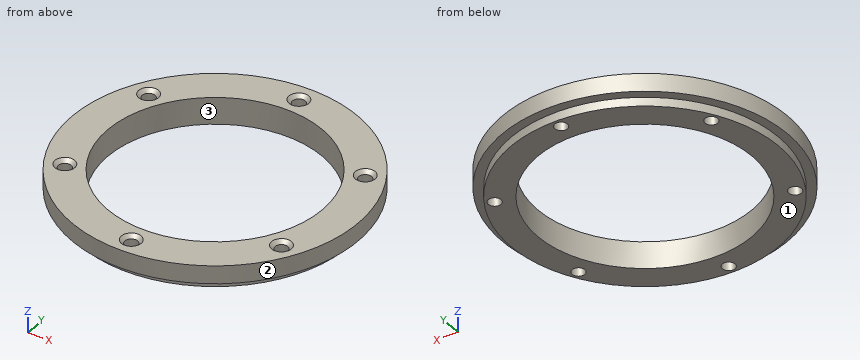
```python
from build123d import *

# Parameters (mm, degrees)
SKETCH1_R                       = 25.4
SKETCH1_R_2                     = 19.05
BOSS_EXTRUDE1_DEPTH             = 4.7625
F_4_40_TAPPED_HOLE1_D           = 2.2606
F_4_40_TAPPED_HOLE1_DEPTH       = 7.62
F_4_40_TAPPED_HOLE1_CSINK_D     = 3.5306
F_4_40_TAPPED_HOLE1_CSINK_ANGLE = 90
F_4_40_TAPPED_HOLE1_TIP         = 0.679152758
SKETCH5_OUTSIDE_W               = 67.2
SKETCH5_OUTSIDE_H               = 67.2
SKETCH5_OUTSIDE_R               = 23.8125
CUT_EXTRUDE1_DEPTH              = 1.5748


with BuildPart() as part:
    # Sketch1 → Boss-Extrude1 (new body)
    with BuildSketch(Plane.XY):
        with Locations(Location((0, 0, 0), (0, 0, 180))):
            Circle(SKETCH1_R)
        with Locations(Location((0, 0, 0), (0, 0, 180))):
            Circle(SKETCH1_R_2, mode=Mode.SUBTRACT)
    extrude(amount=BOSS_EXTRUDE1_DEPTH)

    # #4-40 Tapped Hole1
    with Locations(Plane.XY.offset(4.7625)):
        with Locations((0, 22.225), (-19.247414599, 11.1125), (19.247414599, 11.1125), (19.247414599, -11.1125), (0, -22.225), (-19.247414599, -11.1125)):
            CounterSinkHole(F_4_40_TAPPED_HOLE1_D / 2, F_4_40_TAPPED_HOLE1_CSINK_D / 2, depth=F_4_40_TAPPED_HOLE1_DEPTH, counter_sink_angle=F_4_40_TAPPED_HOLE1_CSINK_ANGLE)
            with Locations((0, 0, -(F_4_40_TAPPED_HOLE1_DEPTH + F_4_40_TAPPED_HOLE1_TIP / 2))):  # 118° drill point
                Cone(0, F_4_40_TAPPED_HOLE1_D / 2, F_4_40_TAPPED_HOLE1_TIP, mode=Mode.SUBTRACT)

    # Sketch5 outside → Cut-Extrude1 (cut)
    with BuildSketch(Plane(origin=(0, 0, 0), x_dir=(-1, 0, 0), z_dir=(0, 0, -1))):
        Rectangle(SKETCH5_OUTSIDE_W, SKETCH5_OUTSIDE_H)
        Circle(SKETCH5_OUTSIDE_R, mode=Mode.SUBTRACT)
    extrude(amount=-CUT_EXTRUDE1_DEPTH, mode=Mode.SUBTRACT)


solid = part.part
```
The listing builds one solid part. Answer for the finished solid, in the listing's coordinates (mm). Face numbers are marked on the shaded views. Round coordinates to 2 decimals unless told otherwise and drop trailing zeros. Loops run counter-clockwise (first coordinate to the right, second up) from the corner with the lowest first, then second, coordinate; pieces in that order, holes last. Notation, with made-up numbers: (-31, 44.25) -> (23, 44.25) arc R14 cw to (23, 71.25) -> close; hole circle Ø5 at (70, 86). An arc over 180 degrees is marked (long way). Use one line per item in the form item = value.
1. The part is cut by section D-D on z = 2.4. Give the number of separate pieces and of enclosed holes in the cut face, and give its area (3 significant figures).
Answer key:
separate_pieces = 1
enclosed_holes = 7
area = 863 mm²
2. The part is cut by section A-A on x = 0. Determine the outline of the cut face in (y, z).
Answer key:
outline = (-25.4, 1.57) -> (-23.81, 1.57) -> (-23.81, 0) -> (-23.36, 0) -> (-23.36, 4.13) -> (-23.99, 4.76) -> (-25.4, 4.76) -> close; (-21.09, 0) -> (-19.05, 0) -> (-19.05, 4.76) -> (-20.46, 4.76) -> (-21.09, 4.13) -> close; (19.05, 0) -> (21.09, 0) -> (21.09, 4.13) -> (20.46, 4.76) -> (19.05, 4.76) -> close; (23.36, 0) -> (23.81, 0) -> (23.81, 1.57) -> (25.4, 1.57) -> (25.4, 4.76) -> (23.99, 4.76) -> (23.36, 4.13) -> close
3. A flat-ended cylindrical pin translates along its axis: pin 1 Ø1.5 at (x, z) = (19.5, 1.5) entering from -Y. Find the tip coordinate at first contact, or state that the pin passes through.
Answer key:
pin_1 = -17.13
4. The part is cut by section C-C on x = 7.5. Determine the outline of the cut face in (y, z), and give its area (3 significant figures).
Answer key:
outline = (-24.27, 1.57) -> (-22.6, 1.57) -> (-22.6, 0) -> (-17.51, 0) -> (-17.51, 4.76) -> (-24.27, 4.76) -> close; (17.51, 0) -> (22.6, 0) -> (22.6, 1.57) -> (24.27, 1.57) -> (24.27, 4.76) -> (17.51, 4.76) -> close
area = 59.1 mm²
5. For a pull along X with two mould halves and no side action, classify the marked faces 1, 2 and 3 as released by +X, released by -X, zero draft, split by the parting line, or undercut.
Answer key:
face_1 = zero draft
face_2 = split by the parting line
face_3 = undercut
6. The part is cut by section B-B on y = 0. Determine the outline of the cut face in (x, z), and give its area (3 significant figures).
Answer key:
outline = (-25.4, 1.57) -> (-23.81, 1.57) -> (-23.81, 0) -> (-19.05, 0) -> (-19.05, 4.76) -> (-25.4, 4.76) -> close; (19.05, 0) -> (23.81, 0) -> (23.81, 1.57) -> (25.4, 1.57) -> (25.4, 4.76) -> (19.05, 4.76) -> close
area = 55.5 mm²
7. Find the intervals of material crossed by probe 1 along Y at (x, z) = (0, 3.05); probe 2 along X at (y, z) = (12, 2.1); probe 3 along Y at (x, z) = (-15, 2.2), in increasing order. Write a range as [from, to].
Answer key:
probe_1 = [-25.4, -23.36], [-21.09, -19.05], [19.05, 21.09], [23.36, 25.4]
probe_2 = [-22.39, -19.95], [-18.55, -14.8], [14.8, 18.55], [19.95, 22.39]
probe_3 = [-20.5, -11.74], [11.74, 20.5]
